Here's how the part is built. I have some questions about the finished solid (model axes, mm). A direction names the side the tool comes from. Coordinates: 2 decimals unless noted, no trailing zeros. Write each loop counter-clockwise with the first axis right and the second up, starting at its lowest first coordinate (ties: lowest second). Pieces come first, ordered by that corner, then holes.
```python
from build123d import *

# Parameters (mm, degrees)
F0_R      = 27.94
F1_DEPTH  = 50.8
F2_R      = 12.7
F3_DEPTH  = 114.3
F6_R      = 8.0768917326
F7_DEPTH  = 97.32637
F9_D      = 20.32
F9_DEPTH  = 127
F9_TIP    = 6.1047438893
F11_D     = 50.8
F11_DEPTH = 127
F11_TIP   = 15.2618597233
F13_D     = 12.7
F13_DEPTH = 93.98
F13_TIP   = 3.8154649308


with BuildPart() as f1:
    # F0 (on Front) → F1 (new body, symmetric)
    with BuildSketch(Plane.XZ):
        Circle(F0_R)
    extrude(amount=F1_DEPTH, both=True)

    # F2 (on Right) → F3 (join)
    with BuildSketch(Plane.YZ):
        with Locations((29.3527785689, 0)):
            Circle(F2_R)
    extrude(amount=F3_DEPTH)

    # F6 (on face) → F7 (join)
    with BuildSketch(Plane(origin=(-14.9178076535, -14.9178076535, 0), x_dir=(-0.7071067812, 0.7071067812, 0), z_dir=(0.7071067812, 0.7071067812, 0))):
        with Locations((-35.2585986257, 0)):
            Circle(F6_R)
    extrude(amount=F7_DEPTH)

    # F9
    with Locations(Plane.YZ.offset(114.3)):
        with Locations((29.3527785689, 0)):
            Hole(F9_D / 2, depth=F9_DEPTH)
            with Locations((0, 0, -(F9_DEPTH + F9_TIP / 2))):  # 118° drill point
                Cone(0, F9_D / 2, F9_TIP, mode=Mode.SUBTRACT)

    # F11
    with Locations(Plane.XZ.offset(50.8)):
        with Locations((0, 0)):
            Hole(F11_D / 2, depth=F11_DEPTH)
            with Locations((0, 0, -(F11_DEPTH + F11_TIP / 2))):  # 118° drill point
                Cone(0, F11_D / 2, F11_TIP, mode=Mode.SUBTRACT)

    # F13
    with Locations(Plane(origin=(-14.9178076535, -14.9178076535, 0), x_dir=(-0.7071067812, 0.7071067812, 0), z_dir=(-0.7071067812, -0.7071067812, 0))):
        with Locations((-34.8447375, 0)):
            Hole(F13_D / 2, depth=F13_DEPTH)
            with Locations((0, 0, -(F13_DEPTH + F13_TIP / 2))):  # 118° drill point
                Cone(0, F13_D / 2, F13_TIP, mode=Mode.SUBTRACT)


solid = f1.part
```
1) Imagine slicing it at B-B on z = 3.5. Please give me the cut outline in (x, y), then the cut area to 3 significant figures.
Values follow:
outline: (-27.72, -50.8) - (-25.16, -50.8) - (-25.16, 50.8) - (-27.72, 50.8) - close; (25.16, -50.8) - (27.72, -50.8) - (27.72, -32.44) - (77.3, 17.14) - (114.3, 17.14) - (114.3, 19.81) - (76.59, 19.81) - (25.16, -31.61) - close; (25.16, -16.63) - (61.6, 19.81) - (25.16, 19.81) - close; (25.16, 38.89) - (114.3, 38.89) - (114.3, 41.56) - (27.72, 41.56) - (27.72, 50.8) - (25.16, 50.8) - close; hole (27.72, -11.85) - (56.71, 17.14) - (27.72, 17.14) - close
area: 1,080 mm2
2) We'd pull the mould along X, two halves only. Please class faces 1 (the face through (-24.227, 0.711, 7.629)), 2 (the face through (114.3, 24, 9)), 3 (the face through (6, 50.8, -25)): pulls with the +X half, pulls with the -X half, needs draft (parallel to the pull), parting line crosses it, or undercut.
Values follow:
face 1: undercut
face 2: pulls with the +X half
face 3: needs draft
3) On a 3-axis mill with a long thin cutter (end or side, diameter ignored), from which of +Z, -Z, +X, -X, +Y, -Y can I reach the whole of each face in a straight line? I mean faces 4 (the face through (68.153, 39.503, 0.447)), 5 (the face through (51.58, -6.26, -1.91)). Say none if no direction works.
Values follow:
face 4: +X
face 5: none
4) Will these pins go through, and if not, where does the flat tip stop? pin 1 (2 mm diameter, centred on y = 7.5, z = -14.5, fed in from +X); pin 2 (3 mm diameter, centred on x = 66, y = 15.5, fed in from +Z); pin 3 (8 mm diameter, centred on y = -6.5, z = 16, fed in from -X); pin 4 (12 mm diameter, centred on x = 90.5, z = 20.5, fed in from +Y).
Values follow:
pin 1: stops at x = 24.46
pin 2: stops at z = 8.08
pin 3: stops at x = -25.23
pin 4: passes through
5) I need wall thicknesses on probe 1 along Y at (x, z) = (89.5, 0); probe 2 along Y at (x, z) = (58, 0); probe 3 along Z at (x, y) = (0, -16.5). Which ranges of each line are inside material? Lowest first, please.
Values follow:
probe 1: y = 16.65 to 19.19, 39.51 to 42.05
probe 2: y = -3.29 to -0.26, 17.7 to 19.19, 39.51 to 42.05
probe 3: z = -27.94 to -25.4, 25.4 to 27.94
6) Imagine slicing it at A-A on x = 0. Please give me the cut outline in (y, z).
Values follow:
outline: (-50.8, -27.94) - (50.8, -27.94) - (50.8, -25.4) - (-50.8, -25.4) - close; (-50.8, 25.4) - (50.8, 25.4) - (50.8, 27.94) - (-50.8, 27.94) - close
7) Imagine slicing it at C-C on z = 19. Please give me the cut outline in (x, y), then the cut area to 3 significant figures.
Values follow:
outline: (-20.49, -50.8) - (-16.86, -50.8) - (-16.86, 50.8) - (-20.49, 50.8) - close; (16.86, -50.8) - (20.49, -50.8) - (20.49, 50.8) - (16.86, 50.8) - close
area: 737 mm2
8) Imagine slicing it at D-D on y = -35. Please give me the cut outline in (x, z), then the cut area to 3 significant figures.
Values follow:
outline: circle Ø55.88 at (0, 0); hole circle Ø50.8 at (0, 0)
area: 426 mm2
